from build123d import *

# Parameters (mm, degrees)
SKETCH_1_W          = 72
SKETCH_1_H          = 35
EXTRUDE_1_DEPTH     = 15
SKETCH_2_W          = 30
SKETCH_2_H          = 2.549015657
EXTRUDE_2_DEPTH     = 16
SKETCH_3_W          = 30
SKETCH_3_H          = 13
EXTRUDE_3_DEPTH     = 18
SKETCH_4_W          = 26
SKETCH_4_H          = 11
CUT_EXTRUDE_1_DEPTH = 6
FILLET_1_R          = 4
FILLET_3_R          = 4
FILLET_2_R          = 1


with BuildPart() as part:
    # ｽｹｯﾁ1 → ﾎﾞｽ - 押し出し1 (new body)
    with BuildSketch(Plane.XY):
        with Locations((36, 17.5)):
            Rectangle(SKETCH_1_W, SKETCH_1_H)
    extrude(amount=EXTRUDE_1_DEPTH)

    # ｽｹｯﾁ2 → ﾎﾞｽ - 押し出し2 (add)
    with BuildSketch(Plane(origin=(0, 35, 0), x_dir=(1, 0, 0), z_dir=(0, 1, 0))):
        with Locations((41, -4.274507828)):
            Rectangle(SKETCH_2_W, SKETCH_2_H)
    extrude(amount=EXTRUDE_2_DEPTH)

    # ｽｹｯﾁ3 → ﾎﾞｽ - 押し出し3 (add)
    with BuildSketch(Plane.XY.offset(5.549015657)):
        with Locations((41, 41.5)):
            Rectangle(SKETCH_3_W, SKETCH_3_H)
    extrude(amount=EXTRUDE_3_DEPTH)

    # ｽｹｯﾁ4 → ｶｯﾄ - 押し出し1 (cut)
    with BuildSketch(Plane.XY.offset(23.549015657)):
        with Locations((41, 41.5)):
            Rectangle(SKETCH_4_W, SKETCH_4_H)
    extrude(amount=-CUT_EXTRUDE_1_DEPTH, mode=Mode.SUBTRACT)

    # ﾌｨﾚｯﾄ1
    fillet_1_edges = [part.edges().sort_by_distance(p)[0] for p in [
        (28, 36, 20.549015657),
        (28, 47, 20.549015657),
        (54, 47, 20.549015657),
        (54, 36, 20.549015657),
    ]]
    fillet(fillet_1_edges, radius=FILLET_1_R)

    # ﾌｨﾚｯﾄ3
    fillet_3_edges = [part.edges().sort_by_distance(p)[0] for p in [
        (26, 35, 9),
    ]]
    fillet(fillet_3_edges, radius=FILLET_3_R)

    # ﾌｨﾚｯﾄ2
    fillet_2_edges = [part.edges().sort_by_distance(p)[0] for p in [
        (26, 35, 19.274507829),
        (26, 48, 14.549015657),
        (56, 35, 19.274507829),
        (56, 48, 14.549015657),
        (0, 35, 7.5),
        (72, 35, 7.5),
        (72, 0, 7.5),
        (0, 0, 7.5),
    ]]
    fillet(fillet_2_edges, radius=FILLET_2_R)


solid = part.part
Can you work these out from the model? Positions are in its coordinate system, mm. A direction names the side the tool comes from. Coordinates: 2 decimals unless noted, no trailing zeros. Order: outer loops, then holes, each group sorted by start corner. A loop starts at its lowest first (then second) coordinate and runs counter-clockwise, first axis right, second up. Notation, with made-up numbers: M 36,75.25 L 92,75.25 A20 ccw 92,93.25 Z; hole C 55,67.25 d11. An arc over 180 degrees is marked long. Write item = value, one per line.
(1) I need wall thicknesses on line 1 along X through (y, z) = (40, 22.25); line 2 along Y through (x, z) = (45.5, 21.5); line 3 along Z through (x, y) = (42, 24.5). Which ranges of each line are inside material? Lowest first, please. Write a range as [from, to].
Results are:
line_1 = [26, 28], [54, 56]
line_2 = [35, 36], [47, 48]
line_3 = [0, 15]
(2) Suppose I cut it at C-C on z = 8. Please give me the cut outline in (x, y), plus the area to 3 significant figures.
Results are:
outline = M 0,1 A1 ccw 1,0 L 71,0 A1 ccw 72,1 L 72,34 A1 ccw 71,35 L 56,35 L 56,47 A1 ccw 55,48 L 27,48 A1 ccw 26,47 L 26,39 A4 cw 22,35 L 1,35 A1 ccw 0,34 Z
area = 2,910 mm2
(3) For pin 1 Ø3.5 at (y, z) = (42, 20.5) entering from -X; pin 2 Ø8 at (y, z) = (36.5, 21) entering from +X; pin 3 Ø12 at (y, z) = (44, 10.5) entering from -X; pin 4 Ø12 at (x, z) = (23.5, 4) entering from +Y, each with a flat end and sliding along its axis, tell me the tip position at first contact or that it passes through.
Results are:
pin_1 = 26
pin_2 = 56
pin_3 = 25.87
pin_4 = 51
(4) Suppose I cut it at B-B on x = 47.5. Please give me the cut outline in (y, z).
Results are:
outline = M 0,0 L 35,0 L 35,3 L 51,3 L 51,5.55 L 48,5.55 L 48,23.55 L 47,23.55 L 47,17.55 L 36,17.55 L 36,23.55 L 35,23.55 L 35,15 L 0,15 Z
(5) Suppose I cut it at D-D on y = 24. Please give me the cut outline in (x, z).
Results are:
outline = M 0,0 L 72,0 L 72,15 L 0,15 Z
(6) Suppose I cut it at A-A on z = 21.5. Please give me the cut outline in (x, y), plus the area to 3 significant figures.
Results are:
outline = M 26,36 A1 ccw 27,35 L 55,35 A1 ccw 56,36 L 56,47 A1 ccw 55,48 L 27,48 A1 ccw 26,47 Z; hole M 28,40 A4 ccw 32,36 L 50,36 A4 ccw 54,40 L 54,43 A4 ccw 50,47 L 32,47 A4 ccw 28,43 Z
area = 117 mm2
(7) For faces 4 (the face through (52.797, 37.141, 20.507)), 5 (the face through (41, 48, 14)), 6 (the face through (26, 43, 13)), 7 (the face through (39, 43, 3)), 8 (the face through (41, 35, 19)), which set-ups out of +Z, -Z, +X, -X, +Y, -Y let a thin tool reach every point of the face, with its end or its side?
Results are:
face_4 = +Z
face_5 = +Z, +X, -X, +Y
face_6 = +Z, -X, +Y
face_7 = -Z, +X, -X, +Y
face_8 = +Z, +X, -X, -Y
(8) If we mould it in two halves opening along X, with no side actions, what happens to faces 1 (the face through (41, 47, 21)), 2 (the face through (72, 17, 7)), 3 (the face through (41, 49, 5.549))? For each: pulls with the +X half, pulls with the -X half, needs draft (parallel to the pull), parting line crosses it, or undercut.
Results are:
face_1 = undercut
face_2 = pulls with the +X half
face_3 = needs draft
